For this review, take the finished solid that the model builds, in its own axes (mm). Face numbers are marked on the shaded views. Give positions to 0.01 mm unless a question says otherwise; leave off trailing zeros. Loops run counter-clockwise (first coordinate to the right, second up) from the corner with the lowest first, then second, coordinate; pieces in that order, holes last. Notation, with made-up numbers: (34, -27.5) -> (78, -27.5) arc R33 ccw to (78, 10.5) -> close; hole circle Ø3 at (72.25, -20.75). An arc over 180 degrees is marked (long way). Answer as CSV lines item,"result". Start each with the question number.
Item 1: For L1, parallel to X at y = 7, z = -9; L2, parallel to Z at x = -37.5, y = 3.5; L3, parallel to Y at x = -61, z = -13, list the stretches that pass through material, from the lowest coordinate up. Write a range as from..to.
Item 2: Clearance check with a flat-ended pin moving along its axis: P1, Ø8, axis at x = 51, z = -7, coming from the -Y side. State where the tip first meets the part, or that it passes through.
Item 3: Add section A-A on y = 4. State the section outline as (x, z) points, plus the area to 3 significant figures.
Item 4: The part is to be moulded in two halves that separate along X. For the marked faces 1 and 2, say which applies: +X half, -X half, draft (parallel to the pull), parting line (faces both ways), or undercut.
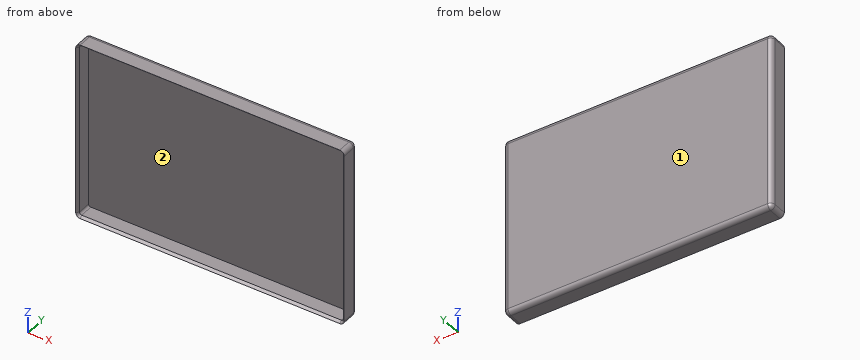
```python
from build123d import *

# Parameters (mm, degrees)
BOSS_EXTRUDE1_DEPTH = 10
SHELL1_T            = -1.25
FILLET1_R           = 2.5
CHAMFER1_SIZE       = 1.25


with BuildPart() as part:
    # Sketch1 → Boss-Extrude1 (new body)
    with BuildSketch(Plane(origin=(0, 0, 0), x_dir=(1, 0, 0), z_dir=(0, 1, 0))):
        with BuildLine():
            Line((-72.5, -50), (72.5, -50))
            ThreePointArc((72.5, -50), (74.267766953, -49.267766953), (75, -47.5))
            Line((75, -47.5), (75, 47.5))
            ThreePointArc((75, 47.5), (74.267766953, 49.267766953), (72.5, 50))
            Line((72.5, 50), (-72.5, 50))
            ThreePointArc((-72.5, 50), (-74.267766953, 49.267766953), (-75, 47.5))
            Line((-75, 47.5), (-75, -47.5))
            ThreePointArc((-75, -47.5), (-74.267766953, -49.267766953), (-72.5, -50))
        make_face()
    extrude(amount=BOSS_EXTRUDE1_DEPTH)

    # Shell1
    shell1_openings = [part.faces().sort_by_distance(p)[0] for p in [
        (0, 0, 0),
    ]]
    offset(amount=SHELL1_T, openings=shell1_openings, kind=Kind.INTERSECTION)

    # Fillet1
    fillet1_edges = [part.edges().sort_by_distance(p)[0] for p in [
        (74.267766953, 10, 49.267766953),
        (75, 10, 0),
        (74.267766953, 10, -49.267766953),
        (0, 10, -50),
        (-74.267766953, 10, -49.267766953),
        (-75, 10, 0),
        (-74.267766953, 10, 49.267766953),
        (0, 10, 50),
    ]]
    fillet(fillet1_edges, radius=FILLET1_R)

    # Chamfer1
    chamfer1_edges = [part.edges().sort_by_distance(p)[0] for p in [
        (-73.383883476, 0, 48.383883476),
        (0, 0, 48.75),
        (73.383883476, 0, 48.383883476),
        (73.75, 0, 0),
        (73.383883476, 0, -48.383883476),
        (0, 0, -48.75),
        (-73.383883476, 0, -48.383883476),
        (-73.75, 0, 0),
    ]]
    chamfer(chamfer1_edges, length=CHAMFER1_SIZE - 0.0001)  # a hair under: the kernel refuses the full size


solid = part.part
```
Computed values:
1,L1,"-75..-73.75, 73.75..75"
1,L2,"-50..-48.75, 48.75..50"
1,L3,"8.75..10"
2,P1,"y = 8.75"
3,outline,"(-75, -47.5) arc R2.5 ccw to (-72.5, -50) -> (72.5, -50) arc R2.5 ccw to (75, -47.5) -> (75, 47.5) arc R2.5 ccw to (72.5, 50) -> (-72.5, 50) arc R2.5 ccw to (-75, 47.5) -> close; hole (-73.75, -47.5) arc R1.25 ccw to (-72.5, -48.75) -> (72.5, -48.75) arc R1.25 ccw to (73.75, -47.5) -> (73.75, 47.5) arc R1.25 ccw to (72.5, 48.75) -> (-72.5, 48.75) arc R1.25 ccw to (-73.75, 47.5) -> close"
3,area,"615 mm²"
4,face 1,"draft"
4,face 2,"undercut"
